from build123d import *

# Parameters (mm, degrees)
SKETCH5_W          = 3.25
SKETCH5_H          = 7.5
CUT_EXTRUDE1_DEPTH = 2.5


with BuildPart() as part:
    # Sketch2 → Revolve1 (revolve)
    with BuildSketch(Plane(origin=(0, 0, 0), x_dir=(0, 0, -1), z_dir=(1, 0, 0))):
        Polygon((34, 0), (44, 0), (44, 2), (35, 2), (35, 14), (34, 14), align=None)
    revolve(axis=Axis((0, 0, 0), (0, 1, 0)))

    # Sketch5 → Cut-Extrude1 (cut)
    with BuildSketch(Plane(origin=(0, 0, 0), x_dir=(-1, 0, 0), z_dir=(0, -1, 0))):
        Polygon((-15.273687611, -33.954802961), (-21.768878139, -30.204802961), (-20.143878139, -27.390220399), (-13.648687611, -31.140220399), align=None)
        with Locations((35.41756575, 0)):
            Rectangle(SKETCH5_W, SKETCH5_H)
        Polygon((-21.768878139, 30.204802961), (-15.273687611, 33.954802961), (-13.648687611, 31.140220399), (-20.143878139, 27.390220399), align=None)
    extrude(amount=-CUT_EXTRUDE1_DEPTH, mode=Mode.SUBTRACT)


solid = part.part
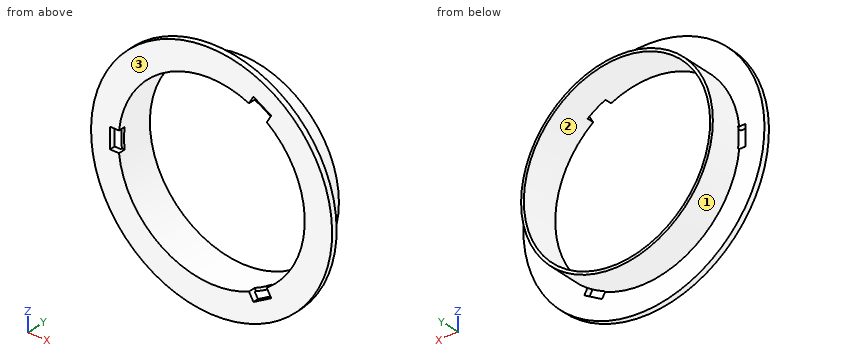
Work out the finished part from the listing and answer in its coordinate system (mm). Face numbers are marked on the shaded views. Give positions to 0.01 mm unless a question says otherwise; leave off trailing zeros. Write each loop counter-clockwise with the first axis right and the second up, starting at its lowest first coordinate (ties: lowest second). Pieces come first, ordered by that corner, then holes.
Q1. The part is cut by section B-B on x = 0. Give the vertices of the cut face in (y, z).
Answer:
outline: (0, -44) - (2, -44) - (2, -35) - (14, -35) - (14, -34) - (0, -34) - close; (0, 34) - (14, 34) - (14, 35) - (2, 35) - (2, 44) - (0, 44) - close
Q2. The part is cut by section A-A on z = 0. Give the vertices of the cut face in (x, y).
Answer:
outline: (-44, 0) - (-37.04, 0) - (-37.04, 2) - (-44, 2) - close; (-35, 2.5) - (-34, 2.5) - (-34, 14) - (-35, 14) - close; (34, 0) - (44, 0) - (44, 2) - (35, 2) - (35, 14) - (34, 14) - close
Q3. The part is cut by section C-C on y = 10.75. Give the vertices of the cut face in (x, z), and give its area (3 significant figures).
Answer:
outline: circle Ø70 at (0, 0); hole circle Ø68 at (0, 0)
area: 217 mm2
Q4. Straight lines are drawn through the part: L1, parallel to Z at x = 0, y = 11; L2, parallel to Y at x = 11, z = 34. For each, find the intervals that lie inside material, in ascending order.
Answer:
L1: z = -35 to -34, 34 to 35
L2: y = 0 to 2
Q5. For a pull along X with two mould halves and no side action, classify the marked faces 1, 2 and 3 as released by +X, released by -X, zero draft, split by the parting line, or undercut.
Answer:
face 1: split by the parting line
face 2: undercut
face 3: zero draft
Q6. Given pin 1 (10 mm diameter, centred on x = 31.5, z = -28, fed in from +Y); pin 2 (1 mm diameter, centred on y = 5.5, z = -30, fed in from +X); pin 3 (1.6 mm diameter, centred on y = 0.5, z = -1.5, fed in from +X), each flat-ended and moving along its own axis, determine where each tip first touches the part or whether it passes through.
Answer:
pin 1: stops at y = 2
pin 2: stops at x = 18.83
pin 3: stops at x = 43.99
Q7. The part is cut by section D-D on x = 18.5. Give the vertices of the cut face in (y, z), and give its area (3 significant figures).
Answer:
outline: (0, -39.92) - (2, -39.92) - (2, -32.09) - (0, -32.09) - close; (0, 32.09) - (2, 32.09) - (2, 39.92) - (0, 39.92) - close; (2.5, -29.71) - (14, -29.71) - (14, -28.53) - (2.5, -28.53) - close; (2.5, 28.53) - (14, 28.53) - (14, 29.71) - (2.5, 29.71) - close
area: 58.6 mm2
